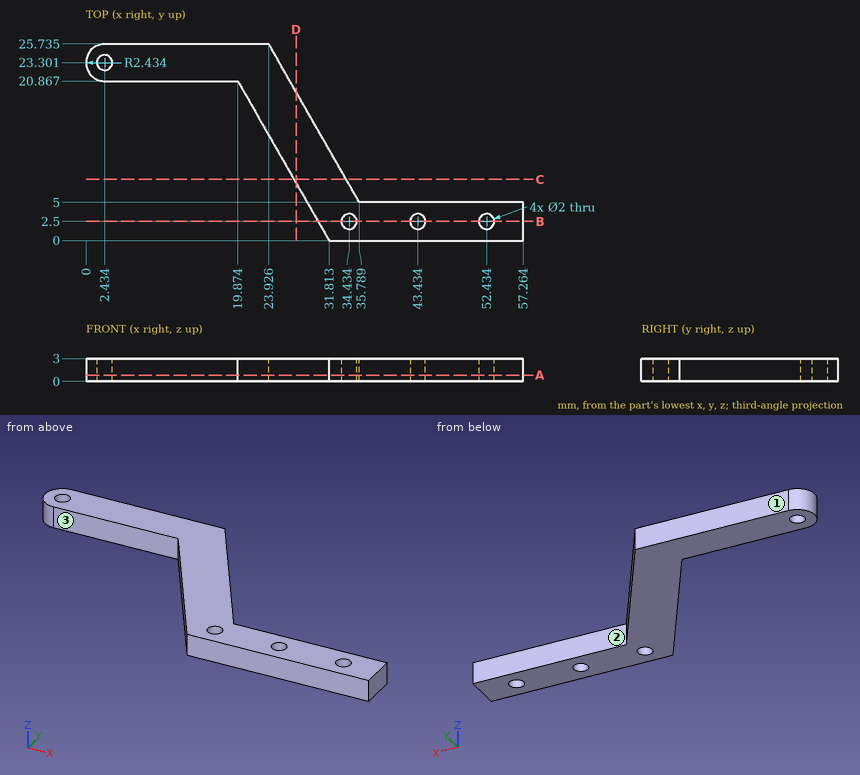
The drawing under review shows one solid part. Ordinate dimensions are in mm from its lowest x, y, z. A direction names the side the tool comes from. Round coordinates to 2 decimals unless told otherwise and drop trailing zeros. Write each loop counter-clockwise with the first axis right and the second up, starting at its lowest first coordinate (ties: lowest second). Pieces come first, ordered by that corner, then holes. Notation, with made-up numbers: (-32, 58.25) -> (-10, 58.25) arc R35 ccw to (-10, 96.25) -> close; hole circle Ø10 at (-4.5, 16.25). An arc over 180 degrees is marked (long way). One line per question, with ' | ' between items. Start each with the question number.
(1) Add section A-A, the plane z = 0.85. Write out the cut boundary in (x, y) (1 decimal).
(2) Add section B-B, the plane y = 2.5. Write out the cut boundary in (x, z).
(3) For line 1 along Y through (x, z) = (43.5, 2.85); line 2 along Y through (x, z) = (55, 1.25); line 3 along Y through (x, z) = (3.5, 2.85) (1 decimal), list the stretches that pass through material, from the lowest coordinate up. Write a range as from..to.
(4) Add section C-C, the plane y = 8. Write out the cut boundary in (x, z) (1 decimal), plus the area to 3 significant figures.
(5) Tool access review of the marked faces 1, 2 and 3: name each direction out of +Z, -Z, +X, -X, +Y, -Y from which nothing blocks a thin tool from reaching the whole face with its end or side.
(6) Add section D-D, the plane x = 27.5. Write out the cut boundary in (y, z).
(7) Insertion check: P1, Ø1.5, axis at x = 14, z = 1.5, coming from the -Y side; P2, Ø1.6, axis at x = 52.43, y = 2.5, coming from the +Z side; P3, Ø0.9, axis at x = 44.5, z = 2, coming from the +Y side. Each pin has a flat end and moves straight along its axis. Give the tip position at first contact, or say it passes through.
Answer list:
1) outline: (2.4, 20.9) -> (19.9, 20.9) -> (31.8, 0) -> (57.3, 0) -> (57.3, 5) -> (35.8, 5) -> (23.9, 25.7) -> (2.4, 25.7) arc R2.4 ccw to start; hole circle Ø2 at (2.4, 23.3); hole circle Ø2 at (34.4, 2.5); hole circle Ø2 at (43.4, 2.5); hole circle Ø2 at (52.4, 2.5)
2) outline: (30.38, 0) -> (33.43, 0) -> (33.43, 3) -> (30.38, 3) -> close; (35.43, 0) -> (42.43, 0) -> (42.43, 3) -> (35.43, 3) -> close; (44.43, 0) -> (51.43, 0) -> (51.43, 3) -> (44.43, 3) -> close; (53.43, 0) -> (57.26, 0) -> (57.26, 3) -> (53.43, 3) -> close
3) line 1: 0..1.5, 3.5..5 | line 2: 0..5 | line 3: 20.9..25.7
4) outline: (27.2, 0) -> (34.1, 0) -> (34.1, 3) -> (27.2, 3) -> close | area: 20.5 mm²
5) face 1: +Z, -Z, +X, -X, +Y | face 2: +Z, -Z, +X, +Y | face 3: +Z, -Z, -X, -Y
6) outline: (7.54, 0) -> (19.49, 0) -> (19.49, 3) -> (7.54, 3) -> close
7) P1: y = 20.87 | P2: through | P3: y = 5
